from build123d import *

# Parameters (mm, degrees)
BOSS_EXTRUDE1_OUTLINE_R   = 5.925
BOSS_EXTRUDE1_OUTLINE_R_2 = 7.5
BOSS_EXTRUDE1_DEPTH       = 45
SKETCH7_W                 = 80
SKETCH7_H                 = 70
BOSS_EXTRUDE2_DEPTH       = 10
SKETCH9_R                 = 1.5
SKETCH9_R_2               = 7.5
SKETCH9_R_3               = 5.925
CUT_EXTRUDE1_DEPTH        = 70.545797618
CUT_EXTRUDE2_DEPTH        = 2.5


# Read off the part's stored shape, not the designer's step: Boss-Extrude1
with BuildPart() as part:
    # Boss-Extrude1 outline → Boss-Extrude1 (new body)
    with BuildSketch(Plane(origin=(0, 0, 0), x_dir=(1, 0, 0), z_dir=(0, 1, 0))):
        with BuildLine():
            Line((2.640241809, 14.738319), (-2.640241809, 14.738319))
            ThreePointArc((-2.640241809, 14.738319), (-3.689731143, 15.03579965), (-4.427017708, 15.839746863))
            ThreePointArc((-4.427017708, 15.839746863), (-19.653719539, 15.760972037), (-10.385543741, 3.679599122))
            ThreePointArc((-10.385543741, 3.679599122), (-9.543059286, 3.663879971), (-8.781822294, 3.302569315))
            Line((-8.781822294, 3.302569315), (-7.664695593, 2.443767924))
            ThreePointArc((-7.664695593, 2.443767924), (-7.049045485, 1.654548176), (-6.892913986, 0.665854179))
            ThreePointArc((-6.892913986, 0.665854179), (0.034441884, -6.92491435), (6.88594973, 0.734384995))
            ThreePointArc((6.88594973, 0.734384995), (7.072047194, 1.812821739), (7.797876599, 2.63186371))
            Line((7.797876599, 2.63186371), (8.985297239, 3.390509952))
            ThreePointArc((8.985297239, 3.390509952), (9.683500506, 3.668968165), (10.435182401, 3.670020805))
            ThreePointArc((10.435182401, 3.670020805), (19.642563369, 15.783654111), (4.427017708, 15.839746863))
            ThreePointArc((4.427017708, 15.839746863), (3.689731143, 15.03579965), (2.640241809, 14.738319))
        make_face()
        Circle(BOSS_EXTRUDE1_OUTLINE_R, mode=Mode.SUBTRACT)
        with Locations((-12.02081528, 12.02081528)):
            Circle(BOSS_EXTRUDE1_OUTLINE_R_2, mode=Mode.SUBTRACT)
        with Locations((12.02081528, 12.02081528)):
            Circle(BOSS_EXTRUDE1_OUTLINE_R_2, mode=Mode.SUBTRACT)
    extrude(amount=BOSS_EXTRUDE1_DEPTH)

    # Sketch7 → Boss-Extrude2 (add)
    # profile 1 of 2: a face of its own
    with BuildSketch(Plane.XZ):
        with Locations((0, -9.851064271)):
            Rectangle(SKETCH7_W, SKETCH7_H)
        with BuildLine():
            ThreePointArc((6.88594973, -0.734384995), (7.072047194, -1.812821739), (7.797876599, -2.63186371))
            Line((7.797876599, -2.63186371), (8.985297239, -3.390509952))
            ThreePointArc((8.985297239, -3.390509952), (9.683500506, -3.668968165), (10.435182401, -3.670020805))
            ThreePointArc((10.435182401, -3.670020805), (19.642563369, -15.783654111), (4.427017708, -15.839746863))
            ThreePointArc((4.427017708, -15.839746863), (3.689731143, -15.03579965), (2.640241809, -14.738319))
            Line((2.640241809, -14.738319), (-2.640241809, -14.738319))
            ThreePointArc((-2.640241809, -14.738319), (-3.689731143, -15.03579965), (-4.427017708, -15.839746863))
            ThreePointArc((-4.427017708, -15.839746863), (-19.653719539, -15.760972037), (-10.385543741, -3.679599122))
            ThreePointArc((-10.385543741, -3.679599122), (-9.543059286, -3.663879971), (-8.781822294, -3.302569315))
            Line((-8.781822294, -3.302569315), (-7.664695593, -2.443767924))
            ThreePointArc((-7.664695593, -2.443767924), (-7.049045485, -1.654548176), (-6.892913986, -0.665854179))
            ThreePointArc((-6.892913986, -0.665854179), (0.034441884, 6.92491435), (6.88594973, -0.734384995))
        make_face(mode=Mode.SUBTRACT)
    # profile 2 of 2: a face of its own
    with BuildSketch(Plane.XZ):
        with Locations((0, -9.851064271)):
            Rectangle(SKETCH7_W, SKETCH7_H)
        with BuildLine():
            ThreePointArc((6.88594973, -0.734384995), (7.072047194, -1.812821739), (7.797876599, -2.63186371))
            Line((7.797876599, -2.63186371), (8.985297239, -3.390509952))
            ThreePointArc((8.985297239, -3.390509952), (9.683500506, -3.668968165), (10.435182401, -3.670020805))
            ThreePointArc((10.435182401, -3.670020805), (19.642563369, -15.783654111), (4.427017708, -15.839746863))
            ThreePointArc((4.427017708, -15.839746863), (3.689731143, -15.03579965), (2.640241809, -14.738319))
            Line((2.640241809, -14.738319), (-2.640241809, -14.738319))
            ThreePointArc((-2.640241809, -14.738319), (-3.689731143, -15.03579965), (-4.427017708, -15.839746863))
            ThreePointArc((-4.427017708, -15.839746863), (-19.653719539, -15.760972037), (-10.385543741, -3.679599122))
            ThreePointArc((-10.385543741, -3.679599122), (-9.543059286, -3.663879971), (-8.781822294, -3.302569315))
            Line((-8.781822294, -3.302569315), (-7.664695593, -2.443767924))
            ThreePointArc((-7.664695593, -2.443767924), (-7.049045485, -1.654548176), (-6.892913986, -0.665854179))
            ThreePointArc((-6.892913986, -0.665854179), (0.034441884, 6.92491435), (6.88594973, -0.734384995))
        make_face(mode=Mode.SUBTRACT)
    extrude(amount=-BOSS_EXTRUDE2_DEPTH)

    # Sketch9 → Cut-Extrude1 (cut, through all)
    with BuildSketch(Plane(origin=(0, 10, 0), x_dir=(-1, 0, 0), z_dir=(0, -1, 0))):
        with Locations(Location((-30, 38.351064271, 0), (0, 0, 90))):
            Circle(SKETCH9_R)
        with Locations(Location((-30, -18.648935729, 0), (0, 0, 90))):
            Circle(SKETCH9_R)
        with Locations(Location((0, -18.648935729, 0), (0, 0, 90))):
            Circle(SKETCH9_R)
        with Locations(Location((30, -18.648935729, 0), (0, 0, 90))):
            Circle(SKETCH9_R)
        with Locations(Location((30, 38.351064271, 0), (0, 0, 90))):
            Circle(SKETCH9_R)
        with Locations(Location((0, 38.351064271, 0), (0, 0, 90))):
            Circle(SKETCH9_R)
        with Locations(Location((-12.02081528, 12.02081528, 0), (0, 0, 90))):
            Circle(SKETCH9_R_2)
        with Locations(Location((12.02081528, 12.02081528, 0), (0, 0, 90))):
            Circle(SKETCH9_R_2)
        with Locations(Location((0, 0, 0), (0, 0, 90))):
            Circle(SKETCH9_R_3)
    extrude(amount=CUT_EXTRUDE1_DEPTH, mode=Mode.SUBTRACT)

    # Sketch10 → Cut-Extrude2 (cut)
    with BuildSketch(Plane(origin=(0, 0, 0), x_dir=(-1, 0, 0), z_dir=(0, 1, 0))):
        with BuildLine():
            Line((-11.434840744, 7.500002811), (-25.410017566, 7.500002811))
            ThreePointArc((-25.410017566, 7.500002811), (-30.80127054, 5.410534914), (-33.376311069, 0.233600397))
            ThreePointArc((-33.376311069, 0.233600397), (-4.816e-06, -33.377128543), (33.376311137, 0.233590765))
            ThreePointArc((33.376311137, 0.233590765), (30.801273238, 5.410526556), (25.410021357, 7.499997189))
            Line((25.410021357, 7.499997189), (11.434844431, 7.499997189))
            ThreePointArc((11.434844431, 7.499997189), (3.362e-06, 13.675), (-11.434840744, 7.500002811))
        make_face()
    extrude(amount=CUT_EXTRUDE2_DEPTH, mode=Mode.SUBTRACT)


solid = part.part
Check sheet for the modelled part. Datum: model origin and axes. Units: mm. A direction names the side the tool comes from. Give positions to 0.01 mm unless a question says otherwise; leave off trailing zeros. Write each loop counter-clockwise with the first axis right and the second up, starting at its lowest first coordinate (ties: lowest second). Pieces come first, ordered by that corner, then holes. Notation, with made-up numbers: (-35, 20) -> (21, 20) arc R8 cw to (21, 30) -> close; hole circle Ø4 at (-34.5, 12.25). An arc over 180 degrees is marked (long way). Write item = value, one per line.
Item 1: Sectioned sample at C-C on x = -30. Record the boundary of the cut face in (y, z).
Output:
outline = (0, -44.85) -> (10, -44.85) -> (10, -39.85) -> (0, -39.85) -> close; (0, -36.85) -> (10, -36.85) -> (10, 17.15) -> (0, 17.15) -> (0, 6.05) -> (2.5, 6.05) -> (2.5, -14.63) -> (0, -14.63) -> close; (0, 20.15) -> (10, 20.15) -> (10, 25.15) -> (0, 25.15) -> close
Item 2: Sectioned sample at D-D on y = 8.5. Count the separate pieces of the cut face and the enclosed holes in it, and give its area (3 significant figures).
Output:
separate_pieces = 1
enclosed_holes = 9
area = 5,090 mm^2
Item 3: Tool access check on faces 1 (the cylindrical face through (31.014, 5.07, 19.754)), 2 (the cylindrical face through (3.7, 27.26, -15.04)), 3 (the flat face through (18, 1, 7.5)), 4 (the cylindrical face through (7.065, 27.255, -1.799)), 5 (the flat face through (-1, 10, -17)). Record the directions out of +Z, -Z, +X, -X, +Y, -Y that give a thin tool (end or side, any length) a straight path to the whole face; none if there is none.
Output:
face_1 = +Y, -Y
face_2 = -Z, +Y
face_3 = -Y
face_4 = +X, +Y
face_5 = +Y
Item 4: Gauge pin test, flat ends, axial feed: pin 1 (3 mm diameter, centred on x = -31, z = 12, fed in from +Y); pin 2 (5 mm diameter, centred on x = 0, y = 29.5, fed in from +Z) (3 decimals); pin 3 (1.5 mm diameter, centred on x = 6.5, z = 7, fed in from -Y). Record the tip position at first contact, or that the pin passes through.
Output:
pin_1 = 10
pin_2 = 6.925
pin_3 = 2.5
Item 5: Release check for a two-part mould opening along Z. For faces 6 (the cylindrical face through (-19.53, 27.26, -16)), 7 (the cylindrical face through (-30.862, 1.232, 5.354)), 8 (the flat face through (-40, 5, -10)), 9 (the cylindrical face through (-7.989, 23.452, -18.345)) record: +Z half, -Z half, draft (parallel to the pull), parting line (faces both ways), or undercut.
Output:
face_6 = parting line
face_7 = undercut
face_8 = draft
face_9 = undercut
Item 6: Scan lines: probe 1 along Z at (x, y) = (0, 3) (3 decimals); probe 2 along Z at (x, y) = (30, 5.25); probe 3 along X at (y, z) = (29.5, -13.5). Record each from-to range of solid material in increasing order. Write a range as from..to.
Output:
probe_1 = -44.851..-39.851, -36.851..-5.925, 5.925..17.149, 20.149..25.149
probe_2 = -44.85..-39.85, -36.85..17.15, 20.15..25.15
probe_3 = -20.39..-19.37, -4.67..4.67, 19.37..20.39
Item 7: Sectioned sample at B-B on z = -10.5. Record the boundary of the cut face in (x, y) (3 decimals), and give its area (3 significant figures).
Output:
outline = (-40, 0) -> (-31.683, 0) -> (-31.683, 2.5) -> (-19.365, 2.5) -> (-19.365, 45) -> (-20.384, 45) -> (-20.384, 10) -> (-40, 10) -> close; (-4.677, 2.5) -> (4.677, 2.5) -> (4.677, 45) -> (-4.677, 45) -> close; (19.365, 2.5) -> (31.683, 2.5) -> (31.683, 0) -> (40, 0) -> (40, 10) -> (20.384, 10) -> (20.384, 45) -> (19.365, 45) -> close
area = 820 mm^2
Item 8: Sectioned sample at A-A on x = 0. Record the boundary of the cut face in (y, z) (3 decimals).
Output:
outline = (0, -44.851) -> (10, -44.851) -> (10, -39.851) -> (0, -39.851) -> close; (0, -36.851) -> (10, -36.851) -> (10, -14.738) -> (45, -14.738) -> (45, -5.925) -> (2.5, -5.925) -> (2.5, -33.377) -> (0, -33.377) -> close; (0, 13.675) -> (2.5, 13.675) -> (2.5, 5.925) -> (45, 5.925) -> (45, 6.925) -> (10, 6.925) -> (10, 17.149) -> (0, 17.149) -> close; (0, 20.149) -> (10, 20.149) -> (10, 25.149) -> (0, 25.149) -> close
